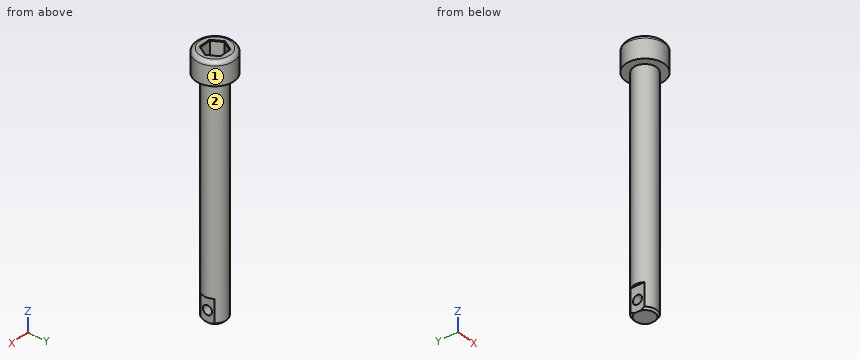
from build123d import *

# Parameters (mm, degrees)
ESQUISSE1_R             = 5
BASE_EXTRUSION_DEPTH    = 6
ENL_V_MAT_EXTRU_1_DEPTH = 4
CONG_1_R                = 1
CHANFREIN3_SIZE         = 0.15
ESQUISSE4_R             = 3
BOSS_EXTRU_1_DEPTH      = 60
CHANFREIN4_SIZE         = 0.5
ESQUISSE5_W             = 1.725795971
ESQUISSE5_H             = 5.746530977
ENL_V_MAT_EXTRU_2_DEPTH = 6.5
ESQUISSE6_W             = 1.6
ESQUISSE6_H             = 6
ENL_V_MAT_EXTRU_3_DEPTH = 6.5
ESQUISSE7_R             = 1.2
ENL_V_MAT_EXTRU_4_DEPTH = 61.661025379


with BuildPart() as part:
    # Esquisse1 → Base-Extrusion (new body)
    with BuildSketch(Plane.XY):
        Circle(ESQUISSE1_R)
    extrude(amount=BASE_EXTRUSION_DEPTH)

    # Esquisse3 → Enlèv. mat.-Extru.1 (cut)
    with BuildSketch(Plane.XY.offset(6)):
        Polygon((-3, 0), (-1.502673246, 2.596530977), (1.502673246, 2.596530977), (3, 0), (1.502673246, -2.596530977), (-1.502673246, -2.596530977), align=None)
    extrude(amount=-ENL_V_MAT_EXTRU_1_DEPTH, mode=Mode.SUBTRACT)

    # Congé1
    cong_1_edges = [part.edges().sort_by_distance(p)[0] for p in [
        (-5, 0, 6),
    ]]
    fillet(cong_1_edges, radius=CONG_1_R)

    # Chanfrein3
    chanfrein3_edges = [part.edges().sort_by_distance(p)[0] for p in [
        (-2.251336623, -1.298265489, 6),
        (0, -2.596530977, 6),
        (2.251336623, -1.298265489, 6),
        (2.251336623, 1.298265489, 6),
        (0, 2.596530977, 6),
        (-2.251336623, 1.298265489, 6),
    ]]
    chamfer(chanfrein3_edges, length=CHANFREIN3_SIZE)

    # Esquisse4 → Boss.-Extru.1 (add)
    with BuildSketch(Plane(origin=(0, 0, 0), x_dir=(-1, 0, 0), z_dir=(0, 0, -1))):
        with Locations(Location((0, 0, 0), (0, 0, 216.869897646))):
            Circle(ESQUISSE4_R)
    extrude(amount=BOSS_EXTRU_1_DEPTH)

    # Chanfrein4
    chanfrein4_edges = [part.edges().sort_by_distance(p)[0] for p in [
        (-2.4, 1.8, -60),
    ]]
    chamfer(chanfrein4_edges, length=CHANFREIN4_SIZE)

    # Esquisse5 → Enlèv. mat.-Extru.2 (cut)
    with BuildSketch(Plane(origin=(0, 0, -60), x_dir=(-1, 0, 0), z_dir=(0, 0, -1))):
        with Locations((-3.262897986, 0.126734511)):
            Rectangle(ESQUISSE5_W, ESQUISSE5_H)
    extrude(amount=-ENL_V_MAT_EXTRU_2_DEPTH, mode=Mode.SUBTRACT)

    # Esquisse6 → Enlèv. mat.-Extru.3 (cut)
    with BuildSketch(Plane(origin=(0, 0, -60), x_dir=(-1, 0, 0), z_dir=(0, 0, -1))):
        with Locations((3.2, 0)):
            Rectangle(ESQUISSE6_W, ESQUISSE6_H)
    extrude(amount=-ENL_V_MAT_EXTRU_3_DEPTH, mode=Mode.SUBTRACT)

    # Esquisse7 → Enlèv. mat.-Extru.4 (cut, through all)
    with BuildSketch(Plane(origin=(2.4, 0, 0), x_dir=(0, 0, -1), z_dir=(1, 0, 0))):
        with Locations((57.030411383, 0)):
            Circle(ESQUISSE7_R)
    extrude(amount=-ENL_V_MAT_EXTRU_4_DEPTH, mode=Mode.SUBTRACT)


solid = part.part
Input: part model. Units: mm. Frame: model coordinates. Face numbers are marked on the shaded views. A direction names the side the tool comes from. Give positions to 0.01 mm unless a question says otherwise; leave off trailing zeros. Order: outer loops, then holes, each group sorted by start corner. A loop starts at its lowest first (then second) coordinate and runs counter-clockwise, first axis right, second up. Notation, with made-up numbers: (37.25, -37.75) - (92.25, -37.75) arc R9 cw to (92.25, -22.75) - close; hole circle Ø6 at (-24, 35.25). An arc over 180 degrees is marked (long way). Answer as a JSON object with one key per item and string values. Group by question number.
Q1. Cut plane A-A, the plane x = 0. Output: boundary loops of the cut face in (y, z).
Q2. First-contact query: pin 1 Ø3 at (y, z) = (0.5, -56) entering from -X; pin 2 Ø6 at (y, z) = (0, -22) entering from -X; pin 3 Ø2 at (y, z) = (3, -42.5) entering from +X; pin 4 Ø1.9 at (y, z) = (0, -57.03) entering from -X. Flat tips, straight axial feed; report the tip coordinate or a pass-through.
Q3. Set-up query: the marked faces 1 and 2. Return all of +Z, -Z, +X, -X, +Y, -Y with unobstructed straight access to the full face (end or side cutting, diameter ignored); none if empty.
Q4. Line query: probe 1 along X at (y, z) = (1.5, -5.5); probe 2 along X at (y, z) = (-0.5, -55); probe 3 along Z at (x, y) = (-2.5, 1.25). Output: solid intervals per line, ascending.
Q5. Cut plane B-B, the plane z = -48.5. Output: boundary loops of the cut face in (x, y), then the cut area to 3 significant figures.
Results:
{
 "1": {"outline": "(-5, 0) - (-3, 0) - (-3, -59.5) - (-2.5, -60) - (2.5, -60) - (3, -59.5) - (3, 0) - (5, 0) - (5, 5) arc R1 ccw to (4, 6) - (2.75, 6) - (2.6, 5.85) - (2.6, 2) - (-2.6, 2) - (-2.6, 5.85) - (-2.75, 6) - (-4, 6) arc R1 ccw to (-5, 5) - close; hole circle Ø2.4 at (0, -57.03)"},
 "2": {"pin 1": "x = -2.4", "pin 2": "x = -3", "pin 3": "x = 2.24", "pin 4": "through"},
 "3": {"face 1": "+Z, -Z", "face 2": "-Z"},
 "4": {"probe 1": "-2.6 to 2.6", "probe 2": "-2.4 to 2.4", "probe 3": "-53.5 to 6"},
 "5": {"outline": "circle Ø6 at (0, 0)", "area": "28.3 mm^2"}
}
